Check sheet for the modelled part. Datum: model origin and axes. Units: mm. Give positions to 0.01 mm unless a question says otherwise; leave off trailing zeros. Order: outer loops, then holes, each group sorted by start corner. A loop starts at its lowest first (then second) coordinate and runs counter-clockwise, first axis right, second up. Notation, with made-up numbers: M 40.5,69.5 L 61.5,69.5 A23 ccw 61.5,79.5 Z; hole C 57.5,-40 d2. An arc over 180 degrees is marked long. Return JSON: item names as keys, results as strings. Group by question number.
from build123d import *

# Parameters (mm, degrees)
CHASSIS_DEPTH       = 6.35
BOSS_EXTRUDE1_DEPTH = 6.35
SKETCH2_R           = 1.5875
SKETCH2_R_2         = 1.5
SKETCH2_R_3         = 1.3716
SKETCH2_R_4         = 2.38125
SKETCH2_W           = 12.7
SKETCH2_H           = 38.1
CUT_EXTRUDE1_DEPTH  = 17.78


with BuildPart() as part:
    # Sketch1 → Chassis (new body)
    with BuildSketch(Plane(origin=(0, 0, 0), x_dir=(1, 0, 0), z_dir=(0, 1, 0))):
        with BuildLine():
            Line((0, 66.173750115), (0, -229.362))
            Line((0, -229.362), (76.2, -229.362))
            Line((76.2, -229.362), (76.2, -191.262))
            Line((76.2, -191.262), (47.117, -191.262))
            Line((47.117, -191.262), (47.117, -116.713))
            Line((47.117, -116.713), (76.2, -116.713))
            Line((76.2, -116.713), (76.2, -42.672))
            Line((76.2, -42.672), (40.132, -42.672))
            Line((40.132, -42.672), (40.132, -13.843))
            Line((40.132, -13.843), (32.512, -13.843))
            Line((32.512, -13.843), (32.512, 14.097))
            Line((32.512, 14.097), (40.132, 14.097))
            Line((40.132, 14.097), (40.132, 42.672))
            Line((40.132, 42.672), (76.2, 42.672))
            Line((76.2, 42.672), (76.2, 49.022))
            ThreePointArc((76.2, 49.022), (39.053241005, 61.832834411), (0, 66.173750115))
        make_face()
    chassis = extrude(amount=CHASSIS_DEPTH)

    # Mirror1: Chassis across plane
    add(chassis.mirror(Plane(origin=(0, 6.35, 0), x_dir=(0, 0, 1), z_dir=(1, 0, 0))))

    # Sketch4 → Boss-Extrude1 (add)
    with BuildSketch(Plane(origin=(0, 6.35, 0), x_dir=(1, 0, 0), z_dir=(0, 1, 0))):
        with BuildLine():
            Line((76.2, -229.362), (-76.2, -229.362))
            ThreePointArc((-76.2, -229.362), (0, -246.518294863), (76.2, -229.362))
        make_face()
    extrude(amount=-BOSS_EXTRUDE1_DEPTH)

    # Sketch2 → Cut-Extrude1 (cut)
    with BuildSketch(Plane(origin=(0, 0, 0), x_dir=(1, 0, 0), z_dir=(0, 1, 0))):
        with Locations((33.096859047, -195.58)):
            Circle(SKETCH2_R)
        with Locations((-18.973140953, -228.6)):
            Circle(SKETCH2_R)
        with Locations((33.096859047, -223.52)):
            Circle(SKETCH2_R)
        with Locations((41.402, -151.796334461)):
            Circle(SKETCH2_R_2)
        with Locations((-26.555704526, 9.169971692)):
            Circle(SKETCH2_R_3)
        with Locations((-20.105647723, 0.999384842)):
            Circle(SKETCH2_R_3)
        with Locations((-27.786476371, -8.040568412)):
            Circle(SKETCH2_R_3)
        with Locations((26.555704526, 9.169971692)):
            Circle(SKETCH2_R_3)
        with Locations((20.105647723, 0.999384842)):
            Circle(SKETCH2_R_3)
        with Locations((27.786476371, -8.040568412)):
            Circle(SKETCH2_R_3)
        with Locations((14.2672, -25.46003476)):
            Circle(SKETCH2_R_4)
        with Locations((14.2672, -35.42953476)):
            Circle(SKETCH2_R_4)
        with Locations((-34.5516, -25.46003476)):
            Circle(SKETCH2_R_4)
        with Locations((-34.5516, -35.42953476)):
            Circle(SKETCH2_R_4)
        with Locations((-41.402, -147.875000023)):
            Circle(SKETCH2_R_2)
        with Locations((-41.402, -166.925000023)):
            Circle(SKETCH2_R_2)
        with Locations((41.402, -166.655334461)):
            Circle(SKETCH2_R_2)
        with BuildLine():
            Line((24.892, -94.488), (24.892, -164.338))
            ThreePointArc((24.892, -164.338), (23.392, -165.838), (21.892, -164.338))
            Line((21.892, -164.338), (21.892, -94.488))
            ThreePointArc((21.892, -94.488), (23.392, -92.988), (24.892, -94.488))
        make_face()
        with BuildLine():
            Line((-3.048, -94.488), (-3.048, -164.338))
            ThreePointArc((-3.048, -164.338), (-4.548, -165.838), (-6.048, -164.338))
            Line((-6.048, -164.338), (-6.048, -94.488))
            ThreePointArc((-6.048, -94.488), (-4.548, -92.988), (-3.048, -94.488))
        make_face()
        with Locations((-22.987, -157.400000023)):
            Rectangle(SKETCH2_W, SKETCH2_H)
    extrude(amount=CUT_EXTRUDE1_DEPTH, mode=Mode.SUBTRACT)


solid = part.part
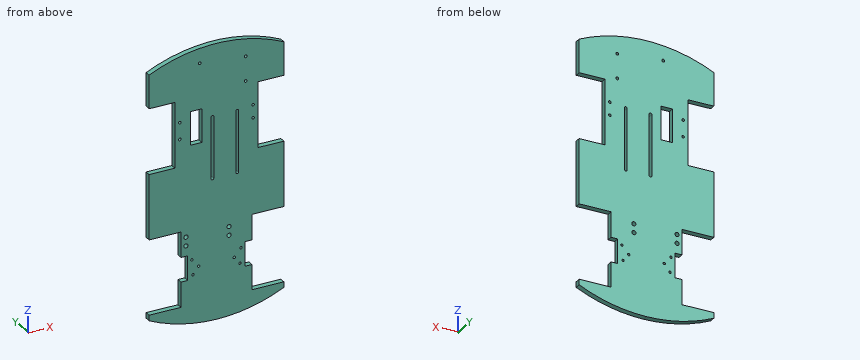
1) Sectioned sample at A-A on z = 121. Record the boundary of the cut face in (x, y), then the cut area to 3 significant figures.
2) Depth check by flat-ended pin: P1, Ø4, axis at x = 2, z = -12.5, coming from the -Y side; P2, Ø3, axis at x = -63, y = 2, coming from the +Z side; P3, Ø1.9, axis at x = -37, y = 2, coming from the +Z side; P4, Ø1.9, axis at x = 36.5, y = 3.5, coming from the +Z side. Enter the tip coordinate at first touch or a pass-through.
3) Material ranges on line 1 along X through (y, z) = (2.5, 104.5); line 2 along X through (y, z) = (3.5, 228.6); line 3 along X through (y, z) = (3.5, 24), recorded low to high.
4) Sectioned sample at D-D on y = 3.75. State how many separate pieces and enclosed holes the cut face has, then the cut area to 3 significant figures.
5) Sectioned sample at B-B on x = -64. Record the boundary of the cut face in (y, z).
6) Sectioned sample at C-C on z = -26.5. Record the boundary of the cut face in (x, y), then the cut area to 3 significant figures.
Reply:
{
 "1": {"outline": "M -47.12,0 L -6.05,0 L -6.05,6.35 L -47.12,6.35 Z; M -3.05,0 L 21.89,0 L 21.89,6.35 L -3.05,6.35 Z; M 24.89,0 L 47.12,0 L 47.12,6.35 L 24.89,6.35 Z", "area": "560 mm^2"},
 "2": {"P1": "y = 0", "P2": "z = 235.54", "P3": "z = 242.83", "P4": "z = 242.93"},
 "3": {"line 1": "-76.2 to -6.05, -3.05 to 21.89, 24.89 to 76.2", "line 2": "-76.2 to -20.56, -17.39 to 76.2", "line 3": "-40.13 to -36.43, -32.67 to 12.39, 16.15 to 40.13"},
 "4": {"separate pieces": "1", "enclosed holes": "20", "area": "34,000 mm^2"},
 "5": {"outline": "M 0,-54.26 L 6.35,-54.26 L 6.35,-42.67 L 0,-42.67 Z; M 0,42.67 L 6.35,42.67 L 6.35,116.71 L 0,116.71 Z; M 0,191.26 L 6.35,191.26 L 6.35,234.6 L 0,234.6 Z"},
 "6": {"outline": "M -40.13,0 L 40.13,0 L 40.13,6.35 L -40.13,6.35 Z", "area": "510 mm^2"}
}
